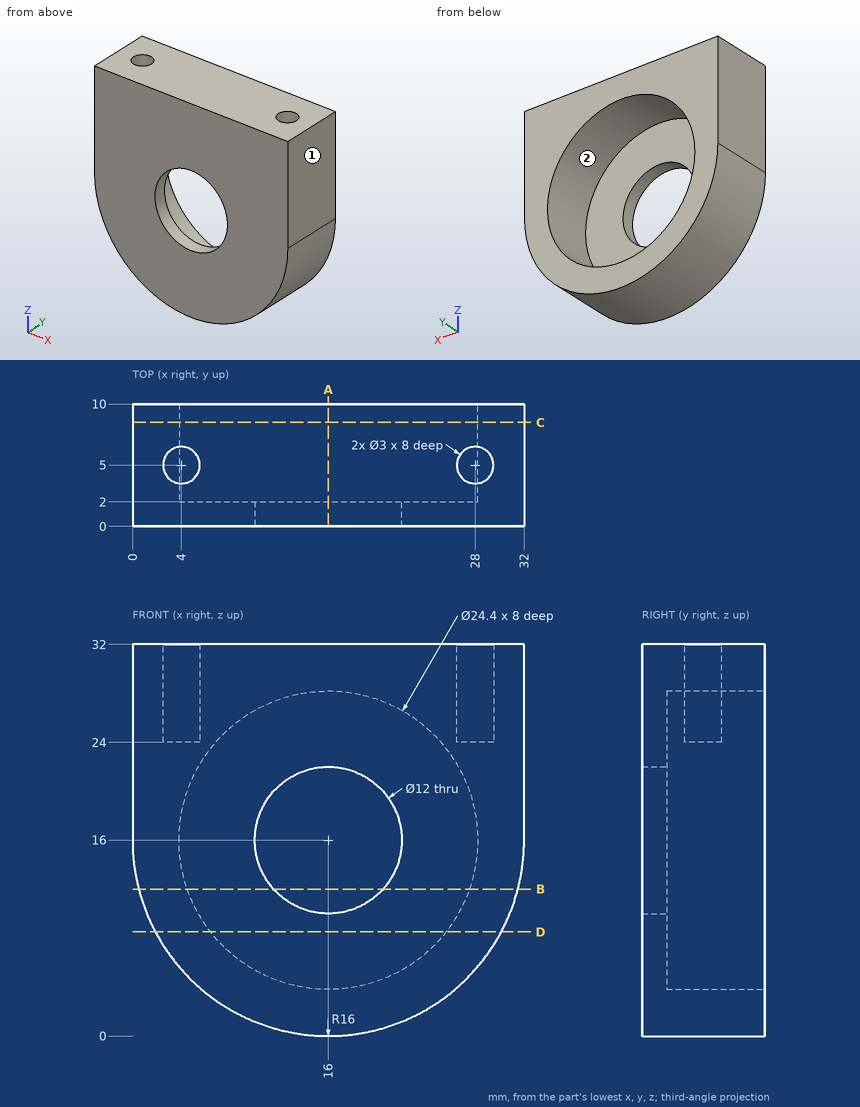
Design review of the part shown in the three views and the two pictorial views. Dimensions are in mm from the part's minimum x, y and z. A direction names the side the tool comes from. Round coordinates to 2 decimals unless told otherwise and drop trailing zeros. Write each loop counter-clockwise with the first axis right and the second up, starting at its lowest first coordinate (ties: lowest second). Pieces come first, ordered by that corner, then holes.
Item 1: For pin 1 Ø19 at (x, z) = (16, 16) entering from -Y; pin 2 Ø2.5 at (x, y) = (4, 5) entering from +Z; pin 3 Ø12 at (x, z) = (15.5, 12.5) entering from +Y, all flat-tipped, find the tip position at first contact; note any pin that passes through.
Item 2: Consider section B-B on z = 12. Give the boundary of the cut face in (x, y).
Item 3: Consider section A-A on x = 16. Give the boundary of the cut face in (y, z).
Item 4: Wall thickness on L1, parallel to Z at x = 16, y = 6.75; L2, parallel to Z at x = 16, y = 1.5; L3, parallel to Y at x = 6, z = 14: over which ranges is each line inside the solid? List them lowest first.
Item 5: Consider section D-D on z = 8.5. Give the boundary of the cut face in (x, y), and give its area (3 significant figures).
Item 6: For the marked faces 1 and 2, list the 3-axis set-ups (+Z, -Z, +X, -X, +Y, -Y) from which the entire face can be reached by the end or side of a thin tool; tool diameter is ignored.
Item 7: Consider section C-C on y = 8.5. Give the boundary of the cut face in (x, z), and give its area (3 significant figures).
Check values:
1. pin 1: stops at y = 0
1. pin 2: stops at z = 24
1. pin 3: stops at y = 2
2. outline: (0.51, 0) - (11.53, 0) - (11.53, 2) - (4.47, 2) - (4.47, 10) - (0.51, 10) - close; (20.47, 0) - (31.49, 0) - (31.49, 10) - (27.53, 10) - (27.53, 2) - (20.47, 2) - close
3. outline: (0, 0) - (10, 0) - (10, 3.8) - (2, 3.8) - (2, 10) - (0, 10) - close; (0, 22) - (2, 22) - (2, 28.2) - (10, 28.2) - (10, 32) - (0, 32) - close
4. L1: z = 0 to 3.8, 28.2 to 32
4. L2: z = 0 to 10, 22 to 32
4. L3: y = 0 to 2
5. outline: (1.87, 0) - (30.13, 0) - (30.13, 10) - (25.62, 10) - (25.62, 2) - (6.38, 2) - (6.38, 10) - (1.87, 10) - close
5. area: 129 mm2
6. face 1: +Z, -Z, +X, +Y, -Y
6. face 2: +Y
7. outline: (0, 16) arc R16 ccw to (32, 16) - (32, 32) - (0, 32) - close; hole circle Ø24.4 at (16, 16)
7. area: 447 mm2
